```python
from build123d import *

# Parameters (mm, degrees)
F0_R     = 7.3867254589
F1_DEPTH = 25
F3_D     = 12
F3_DEPTH = 12
F3_TIP   = 3.6051637142
F4_R     = 5


with BuildPart() as f1:
    # F0 (on Top) → F1 (new body)
    with BuildSketch(Plane.XY):
        Polygon((15.9428178774, -17.4442061965), (-14.0571821226, 34.5173180305), (-44.0571821226, -17.4442061965), align=None)
        with Locations((-21.5571821226, -4.4538251398)):
            Circle(F0_R, mode=Mode.SUBTRACT)
        with Locations((-21.5571821226, -4.4538251398)):
            Circle(F0_R)
    extrude(amount=F1_DEPTH)

    # F3
    with Locations(Plane(origin=(0, 0, 0), x_dir=(1, 0, 0), z_dir=(0, 0, -1))):
        with Locations((-18.1187801063, 2.1665317472)):
            Hole(F3_D / 2, depth=F3_DEPTH)
            with Locations((0, 0, -(F3_DEPTH + F3_TIP / 2))):  # 118° drill point
                Cone(0, F3_D / 2, F3_TIP, mode=Mode.SUBTRACT)

    # F4
    f4_edges = [f1.edges().sort_by_distance(p)[0] for p in [
        (0.942818, 8.536556, 0),
        (-14.057182, -17.444206, 0),
        (-29.057182, 8.536556, 0),
    ]]
    fillet(f4_edges, radius=F4_R)


solid = f1.part
```
Source: CAD feature listing. Evaluate the final solid. Frame: model axes, mm. Round coordinates to 2 decimals unless told otherwise and drop trailing zeros. Loops run counter-clockwise (first coordinate to the right, second up) from the corner with the lowest first, then second, coordinate; pieces in that order, holes last. Notation, with made-up numbers: M -36.5,-37 L 5.5,-37 A10 cw 5.5,-26 Z; hole C 42.5,47 d2. An arc over 180 degrees is marked long. Put each result on its own line as item: value.
(1) Pull-direction query (Y, two-part tool) for faces 1 (the face through (-0.502, 8.187, 1.504)), 2 (the face through (-10, 2, 0)), 3 (the face through (-17.16, -1.77, 14.98)), 4 (the face through (-13.357, 1.484, 6.084)); classes: released by +Y, released by -Y, zero draft, split by the parting line, or undercut.
Solutions:
face 1: released by +Y
face 2: zero draft
face 3: undercut
face 4: undercut
(2) Section A-A, the plane z = 22.5. Return loops of the section in (x, y).
Solutions:
outline: M -44.06,-17.44 L 15.94,-17.44 L -14.06,34.52 Z
(3) First-contact query: pin 1 (3 mm diameter, centred on y = 0.5, z = 5.5, fed in from -X); pin 2 (10 mm diameter, centred on y = -1.5, z = 11, fed in from +X); pin 3 (1 mm diameter, centred on y = 17, z = 4.5, fed in from -X). Flat tips, straight axial feed; report the tip coordinate or a pass-through.
Solutions:
pin 1: x = -34.56
pin 2: x = 9.62
pin 3: x = -24.44
(4) Ray query, line 1 (X direction, y = -5, z = 22); line 2 (X direction, y = -12, z = 17.25); line 3 (Y direction, x = -39, z = 8.25). Return the intervals inside material, ascending. Write a range as [from, to].
Solutions:
line 1: [-36.87, 8.76]
line 2: [-40.91, 12.8]
line 3: [-17.44, -8.68]
(5) Section B-B, the plane z = 13. Return loops of the section in (x, y), and give its area (3 significant figures).
Solutions:
outline: M -44.06,-17.44 L 15.94,-17.44 L -14.06,34.52 Z; hole C -18.12,-2.17 d8.67
area: 1,500 mm²
(6) Section C-C, the plane z = 10. Return loops of the section in (x, y).
Solutions:
outline: M -44.06,-17.44 L 15.94,-17.44 L -14.06,34.52 Z; hole C -18.12,-2.17 d12
